Input: dimensioned drawing with shaded views. Units: mm. Origin: part minimum x, y, z. A direction names the side the tool comes from. Round coordinates to 2 decimals unless told otherwise and drop trailing zeros. Order: outer loops, then holes, each group sorted by start corner. A loop starts at its lowest first (then second) coordinate and runs counter-clockwise, first axis right, second up. Notation, with made-up numbers: M 39.5,49.5 L 46.5,49.5 A11 ccw 46.5,61.5 Z; hole C 71,61 d5. An arc over 180 degrees is marked long. Put each result on its own line as item: value. Start each with the question number.
1) First-contact query: P1, Ø3, axis at x = 5.5, z = 13, coming from the +Y side; P2, Ø3.5, axis at x = 6.5, y = 6.5, coming from the -Z side; P3, Ø1.5, axis at x = 8, z = 4.5, coming from the -Y side; P4, Ø2, axis at y = 3.5, z = 13, coming from the -X side. Flat tips, straight axial feed; report the tip coordinate or a pass-through.
2) Section B-B, the plane x = 9.5. Return loops of the section in (y, z), then the cut area to 3 significant figures.
3) Access query for the marked faces 1, 2, 3, 4 and 5. Directions: +Z, -Z, +X, -X, +Y, -Y. A direction counts if a zero-diameter tool reaches every point of the face in a straight line with its end or side. Return the directions, or none.
4) Section A-A, the plane y = 6.5. Return loops of the section in (x, z).
5) Section C-C, the plane x = 3.25. Return loops of the section in (y, z).
6) Material intervals for probe 1 along Y at (x, z) = (7.5, 4); probe 2 along Z at (x, y) = (11.5, 9); probe 3 along Z at (x, y) = (3, 11), sorted ascending. Write a range as [from, to].
7) Section D-D, the plane z = 6. Return loops of the section in (x, y).
8) Draft query along X for the marked faces 6, 7 and 8. Return one class per face: pulls with the +X half, pulls with the -X half, needs draft (parallel to the pull), parting line crosses it, or undercut.
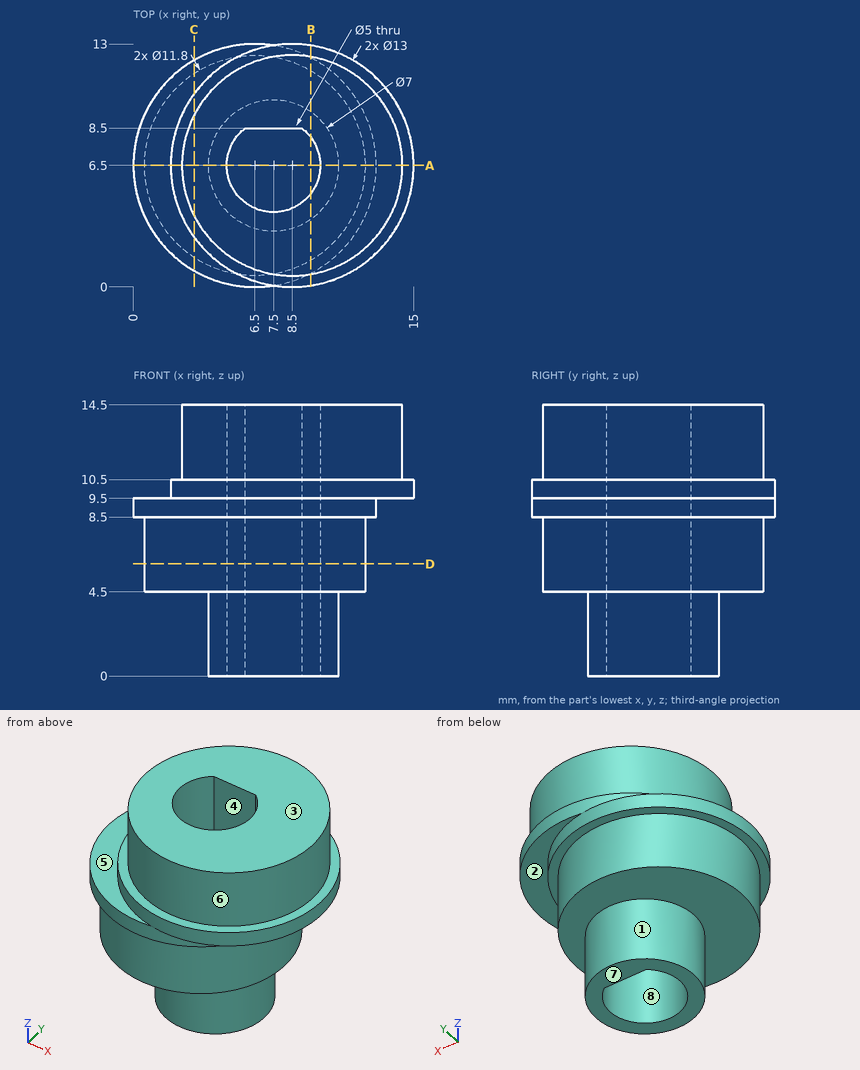
Result sheet:
1. P1: stops at y = 12.21
1. P2: stops at z = 0
1. P3: stops at y = 0.65
1. P4: stops at x = 2.95
2. outline: M 0.08,9.5 L 0.73,9.5 L 0.73,8.5 L 1.42,8.5 L 1.42,4.5 L 3.63,4.5 L 3.63,0 L 5,0 L 5,14.5 L 0.69,14.5 L 0.69,10.5 L 0.08,10.5 Z; M 8,0 L 9.37,0 L 9.37,4.5 L 11.58,4.5 L 11.58,8.5 L 12.27,8.5 L 12.27,9.5 L 12.92,9.5 L 12.92,10.5 L 12.31,10.5 L 12.31,14.5 L 8,14.5 Z
2. area: 93.9 mm2
3. face 1: -Z
3. face 2: -Z, +X
3. face 3: +Z, +X, -X, +Y, -Y
3. face 4: +Z, -Z
3. face 5: +Z, -X
4. outline: M 0,8.5 L 0.6,8.5 L 0.6,4.5 L 4,4.5 L 4,0 L 5,0 L 5,14.5 L 2.6,14.5 L 2.6,10.5 L 2,10.5 L 2,9.5 L 0,9.5 Z; M 10,0 L 11,0 L 11,4.5 L 12.4,4.5 L 12.4,8.5 L 13,8.5 L 13,9.5 L 15,9.5 L 15,10.5 L 14.4,10.5 L 14.4,14.5 L 10,14.5 Z
5. outline: M 0.87,8.5 L 1.58,8.5 L 1.58,4.5 L 11.42,4.5 L 11.42,8.5 L 12.13,8.5 L 12.13,9.5 L 10.33,9.5 L 10.33,10.5 L 9.19,10.5 L 9.19,14.5 L 3.81,14.5 L 3.81,10.5 L 2.67,10.5 L 2.67,9.5 L 0.87,9.5 Z
6. probe 1: y = [3, 4], [8.5, 10]
6. probe 2: z = [4.5, 14.5]
6. probe 3: z = [4.5, 9.5]
7. outline: C 6.5,6.5 d11.8; hole M 6,8.5 A2.5 ccw long 9,8.5 Z
8. face 6: parting line crosses it
8. face 7: needs draft
8. face 8: undercut
